Check sheet for the modelled part. Datum: model origin and axes. Units: mm. Coordinates: 2 decimals unless noted, no trailing zeros. Order: outer loops, then holes, each group sorted by start corner. A loop starts at its lowest first (then second) coordinate and runs counter-clockwise, first axis right, second up.
1. Draft check along X on faces 1 (the flat face through (5.276, 0.986, 42.33)), 2 (the cylindrical face through (-39.64, 1.01, 57.6)). Enter one of: released by +X, released by -X, zero draft, split by the parting line, or undercut.
2. Cross-section at A-A (x = -18). Enter the section's corners in (y, z), then the cut area to 3 significant figures.
3. Thickness scan on line 1 (Z direction, x = -18, y = 0.7); line 2 (X direction, y = 0.5, z = 2.5); line 3 (Z direction, x = 1.5, y = 0.8). Record the ranges inside material, lowest first.
4. Cross-section at C-C (z = 41). Count the separate pieces of the cut face and the enclosed holes in it, then the cut area to 3 significant figures.
5. Cross-section at B-B (z = -29). Enter the section's corners in (x, y), then the cut area to 3 significant figures.
```python
from build123d import *

# Parameters (mm, degrees)
SKETCH_1_W             = 81
SKETCH_1_H             = 117
EXTRUDE_1_DEPTH        = 2
FILLET_2_R             = 3
SKETCH_2_R             = 1.4
SKETCH_2_R_2           = 1.65
CUT_EXTRUDE_1_DEPTH    = 10
CUT_EXTRUDE_2_DEPTH    = 10
FILLET_3_R             = 2
CUT_EXTRUDE_3_DEPTH    = 10
FILLET_4_R             = 2
SKETCH_6_W             = 26
SKETCH_6_H             = 26
CUT_EXTRUDE_4_DEPTH    = 10
FILLET_5_R             = 5
CUT_EXTRUDE_5_DEPTH    = 10
FILLET_6_R             = 2
FILLET_6_OF_MIRROR_1_R = 2
CUT_EXTRUDE_6_DEPTH    = 10
CUT_EXTRUDE_7_DEPTH    = 10
FILLET_7_R             = 2


with BuildPart() as part:
    # 草图1 → 凸台-拉伸1 (new body)
    with BuildSketch(Plane(origin=(0, 0, 0), x_dir=(1, 0, 0), z_dir=(0, 1, 0))):
        Rectangle(SKETCH_1_W, SKETCH_1_H)
    extrude(amount=EXTRUDE_1_DEPTH)

    # 圆角2
    fillet_2_edges = [part.edges().sort_by_distance(p)[0] for p in [
        (40.5, 1, 58.5),
        (-40.5, 1, 58.5),
        (-40.5, 1, -58.5),
        (40.5, 1, -58.5),
    ]]
    fillet(fillet_2_edges, radius=FILLET_2_R)

    # 草图2 → 切除-拉伸1 (cut)
    with BuildSketch(Plane.XZ):
        with Locations((-18.000036, 16.931963864)):
            Circle(SKETCH_2_R)
        with Locations((18.068036136, 16.931963864)):
            Circle(SKETCH_2_R)
        with Locations((-18.000036, 53.000036)):
            Circle(SKETCH_2_R)
        with Locations((17.999928, 52.999964)):
            Circle(SKETCH_2_R)
        with Locations((-18, -18.000036)):
            Circle(SKETCH_2_R)
        with Locations((18, -18)):
            Circle(SKETCH_2_R)
        with Locations((-18.068108136, -53.999964)):
            Circle(SKETCH_2_R)
        with Locations((17.999928, -53.999964)):
            Circle(SKETCH_2_R)
        with Locations((-35, 41)):
            Circle(SKETCH_2_R_2)
        with Locations((35, 41)):
            Circle(SKETCH_2_R_2)
        with Locations((35, -19)):
            Circle(SKETCH_2_R_2)
        with Locations((-35, -19)):
            Circle(SKETCH_2_R_2)
        with Locations((-35, 31)):
            Circle(SKETCH_2_R_2)
        with Locations((-35, -29)):
            Circle(SKETCH_2_R_2)
        with Locations((35, -29)):
            Circle(SKETCH_2_R_2)
        with Locations((35, 31)):
            Circle(SKETCH_2_R_2)
    extrude(amount=-CUT_EXTRUDE_1_DEPTH, mode=Mode.SUBTRACT)

    # 草图4 → 切除-拉伸2 (cut)
    with BuildSketch(Plane.XZ):
        with BuildLine():
            Line((31.5, -58.5), (31.5, -51.5))
            Line((31.5, -51.5), (40.5, -51.5))
            Line((40.5, -51.5), (40.5, -55.5))
            ThreePointArc((40.5, -55.5), (39.621320344, -57.621320344), (37.5, -58.5))
            Line((37.5, -58.5), (31.5, -58.5))
        make_face()
        with BuildLine():
            Line((-37.5, -58.5), (-31.5, -58.5))
            Line((-31.5, -58.5), (-31.5, -51.5))
            Line((-31.5, -51.5), (-40.5, -51.5))
            Line((-40.5, -51.5), (-40.5, -55.5))
            ThreePointArc((-40.5, -55.5), (-39.621320344, -57.621320344), (-37.5, -58.5))
        make_face()
    extrude(amount=-CUT_EXTRUDE_2_DEPTH, mode=Mode.SUBTRACT)

    # 圆角3
    fillet_3_edges = [part.edges().sort_by_distance(p)[0] for p in [
        (31.5, 1, -58.5),
        (31.5, 1, -51.5),
        (40.5, 1, -51.5),
        (-40.5, 1, -51.5),
        (-31.5, 1, -51.5),
        (-31.5, 1, -58.5),
    ]]
    fillet(fillet_3_edges, radius=FILLET_3_R)

    # 草图5 → 切除-拉伸3 (cut)
    with BuildSketch(Plane.XZ):
        Polygon((-12.344679588, 49.465999932), (12.412679725, 49.465999932), (0.034000068, 37.087320275), align=None)
        Polygon((-15.965999932, 48.844679588), (-15.965999932, 21.087320275), (-2.087320275, 34.965999932), align=None)
        Polygon((16.034000068, 48.844679588), (16.034000068, 21.087320275), (2.155320412, 34.965999932), align=None)
        Polygon((12.412679725, 20.465999932), (0.034000068, 32.844679588), (-12.344679588, 20.465999932), align=None)
        Polygon((12.412679725, -21.534036068), (0.034000068, -33.912715725), (-12.344679588, -21.534036068), align=None)
        Polygon((16.034000068, -22.155356412), (2.155320412, -36.034036068), (16.034000068, -49.912715725), align=None)
        Polygon((12.412679725, -50.534036068), (0.034000068, -38.155356412), (-12.344679588, -50.534036068), align=None)
        Polygon((-2.087320275, -36.034036068), (-15.965999932, -49.912715725), (-15.965999932, -22.155356412), align=None)
    extrude(amount=-CUT_EXTRUDE_3_DEPTH, mode=Mode.SUBTRACT)

    # 圆角4
    fillet_4_edges = [part.edges().sort_by_distance(p)[0] for p in [
        (-12.344679588, 1, -21.534036068),
        (12.412679725, 1, -21.534036068),
        (0.034000068, 1, -33.912715725),
        (12.412679725, 1, 20.465999932),
        (-12.344679588, 1, 20.465999932),
        (0.034000068, 1, 32.844679588),
        (2.155320412, 1, 34.965999932),
        (16.034000068, 1, 48.844679588),
        (16.034000068, 1, 21.087320275),
        (-15.965999932, 1, 48.844679588),
        (-2.087320275, 1, 34.965999932),
        (-15.965999932, 1, 21.087320275),
        (-15.965999932, 1, -22.155356412),
        (-2.087320275, 1, -36.034036068),
        (-15.965999932, 1, -49.912715725),
        (16.034000068, 1, -22.155356412),
        (16.034000068, 1, -49.912715725),
        (2.155320412, 1, -36.034036068),
        (12.412679725, 1, -50.534036068),
        (-12.344679588, 1, -50.534036068),
        (0.034000068, 1, -38.155356412),
        (0.034000068, 1, 37.087320275),
        (-12.344679588, 1, 49.465999932),
        (12.412679725, 1, 49.465999932),
    ]]
    fillet(fillet_4_edges, radius=FILLET_4_R)

    # 草图6 → 切除-拉伸4 (cut)
    with BuildSketch(Plane.XZ):
        Rectangle(SKETCH_6_W, SKETCH_6_H)
    extrude(amount=-CUT_EXTRUDE_4_DEPTH, mode=Mode.SUBTRACT)

    # 圆角5
    fillet_5_edges = [part.edges().sort_by_distance(p)[0] for p in [
        (13, 1, 13),
        (13, 1, -13),
        (-13, 1, -13),
        (-13, 1, 13),
    ]]
    fillet(fillet_5_edges, radius=FILLET_5_R)

    # 草图7 → 切除-拉伸5 (cut)
    with BuildSketch(Plane.XZ):
        Polygon((35.5, 12.5), (35.5, -12.5), (18, 0), align=None)
    cut_extrude_5 = extrude(amount=-CUT_EXTRUDE_5_DEPTH, mode=Mode.SUBTRACT)

    # 圆角6
    fillet_6_edges = [part.edges().sort_by_distance(p)[0] for p in [
        (18, 1, 0),
        (35.5, 1, 12.5),
        (35.5, 1, -12.5),
    ]]
    fillet(fillet_6_edges, radius=FILLET_6_R)

    # 镜向1: 切除-拉伸5 across plane
    add(cut_extrude_5.mirror(Plane(origin=(0, 0, 0), x_dir=(0, 0, 1), z_dir=(1, 0, 0))), mode=Mode.SUBTRACT)

    # 圆角6 of 镜向1
    fillet_6_of_mirror_1_edges = [part.edges().sort_by_distance(p)[0] for p in [
        (-18, 1, 0),
        (-35.5, 1, 12.5),
        (-35.5, 1, -12.5),
    ]]
    fillet(fillet_6_of_mirror_1_edges, radius=FILLET_6_OF_MIRROR_1_R)

    # 草图8 → 切除-拉伸6 (cut)
    with BuildSketch(Plane.XZ):
        Polygon((-24.241669751, -34.5), (-31.74722325, -34.5), (-35.5, -41), (-31.74722325, -47.5), (-24.241669751, -47.5), (-20.488893001, -41), align=None)
        Polygon((31.74722325, -34.5), (24.241669751, -34.5), (20.488893001, -41), (24.241669751, -47.5), (31.74722325, -47.5), (35.5, -41), align=None)
    extrude(amount=-CUT_EXTRUDE_6_DEPTH, mode=Mode.SUBTRACT)

    # 草图9 → 切除-拉伸7 (cut)
    with BuildSketch(Plane.XZ):
        Polygon((-19.965999932, 47.5), (-19.965999932, 24.5), (-32, 36), align=None)
        Polygon((32.074154001, 36.105834574), (20.002229418, 47.566017579), (20.078209775, 24.566143079), align=None)
    extrude(amount=-CUT_EXTRUDE_7_DEPTH, mode=Mode.SUBTRACT)

    # 圆角7
    fillet_7_edges = [part.edges().sort_by_distance(p)[0] for p in [
        (-24.241669751, 1, -34.5),
        (-20.488893001, 1, -41),
        (-24.241669751, 1, -47.5),
        (-31.74722325, 1, -47.5),
        (-35.5, 1, -41),
        (-31.74722325, 1, -34.5),
        (31.74722325, 1, -34.5),
        (35.5, 1, -41),
        (31.74722325, 1, -47.5),
        (24.241669751, 1, -47.5),
        (20.488893001, 1, -41),
        (24.241669751, 1, -34.5),
        (-32, 1, 36),
        (-19.965999932, 1, 47.5),
        (-19.965999932, 1, 24.5),
        (32.074154001, 1, 36.105834574),
        (20.078209775, 1, 24.566143079),
        (20.002229418, 1, 47.566017579),
    ]]
    fillet(fillet_7_edges, radius=FILLET_7_R)


solid = part.part
```
Data:
1. face 1: undercut
1. face 2: released by -X
2. outline: (0, -58.5) - (2, -58.5) - (2, -55.4) - (0, -55.4) - close; (0, -52.6) - (2, -52.6) - (2, -19.4) - (0, -19.4) - close; (0, -16.6) - (2, -16.6) - (2, 15.53) - (0, 15.53) - close; (0, 18.33) - (2, 18.33) - (2, 51.6) - (0, 51.6) - close; (0, 54.4) - (2, 54.4) - (2, 58.5) - (0, 58.5) - close
2. area: 212 mm2
3. line 1: z = -58.5 to -55.4, -52.6 to -19.4, -16.6 to 15.53, 18.33 to 51.6, 54.4 to 58.5
3. line 2: x = -40.5 to -35.5, -21.5 to -13, 13 to 21.5, 35.5 to 40.5
3. line 3: z = -58.5 to -50.53, -39.62 to -32.45, -21.53 to -13, 13 to 20.47, 31.38 to 38.55, 49.47 to 58.5
4. separate pieces: 8
4. enclosed holes: 0
4. area: 74.4 mm2
5. outline: (-40.5, 0) - (-36.65, 0) - (-36.65, 2) - (-40.5, 2) - close; (-33.35, 0) - (-15.97, 0) - (-15.97, 2) - (-33.35, 2) - close; (-9.12, 0) - (-4.88, 0) - (-4.88, 2) - (-9.12, 2) - close; (4.95, 0) - (9.19, 0) - (9.19, 2) - (4.95, 2) - close; (16.03, 0) - (33.35, 0) - (33.35, 2) - (16.03, 2) - close; (36.65, 0) - (40.5, 0) - (40.5, 2) - (36.65, 2) - close
5. area: 102 mm2
